from build123d import *

# Parameters (mm, degrees)
F0_W         = 100
F0_H         = 40
F1_DEPTH     = 10
F3_DEPTH     = 8.82827
F4_W         = 40
F4_H         = 3
F5_DEPTH     = 40.001
F6_R         = 2.25
F7_DEPTH     = 40.001
F8_R         = 4.5
F9_DEPTH     = 5.7
F10_T1_DEPTH = 40
F10_T3_DEPTH = 50
F10_T5_DEPTH = 50
F10_T7_DEPTH = 50
F10_T9_DEPTH = 50
F11_T1_DEPTH = 40
F12_R        = 3


# Not quite as in the source:
# - a fillet or chamfer that OpenCascade refuses, or shapes differently, is made with other operations: its cross-section is extruded or revolved along the edge and cut away or added


with BuildPart() as f1:
    # F0 (on Top) → F1 (new body)
    with BuildSketch(Plane.XY):
        with Locations((-50, 20)):
            Rectangle(F0_W, F0_H)
    extrude(amount=F1_DEPTH)

    # F2 (on face) → F3 (join)
    with BuildSketch(Plane.XZ):
        with BuildLine():
            ThreePointArc((-30, 35), (-50, 55), (-70, 35))
            Line((-70, 35), (-70, 0))
            Line((-70, 0), (-30, 0))
            Line((-30, 0), (-30, 35))
        make_face()
    extrude(amount=-F3_DEPTH)

    # F4 (on Front) → F5 (cut, through all)
    with BuildSketch(Plane.XZ):
        with Locations((-50, 1.5)):
            Rectangle(F4_W, F4_H)
    extrude(amount=-F5_DEPTH, mode=Mode.SUBTRACT)

    # F6 (on face) → F7 (cut, through all)
    with BuildSketch(Plane.XZ):
        with Locations((-50, 35)):
            Circle(F6_R)
    extrude(amount=-F7_DEPTH, mode=Mode.SUBTRACT)

    # F8 (on face) → F9 (cut)
    with BuildSketch(Plane.XZ):
        with Locations((-50, 35)):
            Circle(F8_R)
    extrude(amount=-F9_DEPTH, mode=Mode.SUBTRACT)

    # F10: fillet of radius 8 on 5 edges, made by hand

    # F10_s2 → F10_t1 (join)
    with BuildSketch(Plane.XZ.offset(-40)):
        with BuildLine():
            ThreePointArc((-36.2449979984, 3), (-32.7808963833, 2.2111025509), (-30, 0))
            Line((-30, 0), (-30, 3))
            Line((-30, 3), (-36.2449979984, 3))
        make_face()
    extrude(amount=F10_T1_DEPTH)

    # F10_s4 → F10_t3 (cut)
    with BuildSketch(Plane.XY.offset(-20)):
        with BuildLine():
            ThreePointArc((-92, 0), (-97.6568542495, 2.3431457505), (-100, 8))
            Line((-100, 8), (-100, 0))
            Line((-100, 0), (-92, 0))
        make_face()
    extrude(amount=F10_T3_DEPTH, mode=Mode.SUBTRACT)

    # F10_s6 → F10_t5 (cut)
    with BuildSketch(Plane.XY.offset(-20)):
        with BuildLine():
            ThreePointArc((-8, 0), (-2.3431457505, 2.3431457505), (0, 8))
            Line((0, 8), (0, 0))
            Line((0, 0), (-8, 0))
        make_face()
    extrude(amount=F10_T5_DEPTH, mode=Mode.SUBTRACT)

    # F10_s8 → F10_t7 (cut)
    with BuildSketch(Plane.XY.offset(-20)):
        with BuildLine():
            ThreePointArc((-100, 32), (-97.6568542495, 37.6568542495), (-92, 40))
            Line((-92, 40), (-100, 40))
            Line((-100, 40), (-100, 32))
        make_face()
    extrude(amount=F10_T7_DEPTH, mode=Mode.SUBTRACT)

    # F10_s10 → F10_t9 (cut)
    with BuildSketch(Plane.XY.offset(-20)):
        with BuildLine():
            ThreePointArc((-8, 40), (-2.3431457505, 37.6568542495), (0, 32))
            Line((0, 32), (0, 40))
            Line((0, 40), (-8, 40))
        make_face()
    extrude(amount=F10_T9_DEPTH, mode=Mode.SUBTRACT)

    # F11: fillet of radius 8 on 1 edges, made by hand

    # F11_s2 → F11_t1 (join)
    with BuildSketch(Plane.XZ.offset(-40)):
        with BuildLine():
            ThreePointArc((-70, 0), (-67.2191036167, 2.2111025509), (-63.7550020016, 3))
            Line((-63.7550020016, 3), (-70, 3))
            Line((-70, 3), (-70, 0))
        make_face()
    extrude(amount=F11_T1_DEPTH)

    # F12
    f12_edges = [f1.edges().sort_by_distance(p)[0] for p in [
        (-50, 8.82827, 55),
        (-30, 8.82827, 22.5),
        (-70, 8.82827, 22.5),
    ]]
    fillet(f12_edges, radius=F12_R)


solid = f1.part
Input: part model. Units: mm. Frame: model coordinates. A direction names the side the tool comes from. Give positions to 0.01 mm unless a question says otherwise; leave off trailing zeros. Write each loop counter-clockwise with the first axis right and the second up, starting at its lowest first coordinate (ties: lowest second). Pieces come first, ordered by that corner, then holes.
Q1. Material intervals for probe 1 along Z at (x, y) = (-50, 2.1); probe 2 along Z at (x, y) = (-90, 35.5); probe 3 along Y at (x, z) = (-51.5, 37), sorted ascending.
Q2. First-contact query: P1, Ø1, axis at y = 4.5, z = 27.5, coming from the +X side; P2, Ø6.5, axis at y = 4, z = 19.5, coming from the -X side; P3, Ø1.5, axis at x = -15, y = 11, coming from the +Z side; P4, Ø7, axis at x = -50.5, z = 34, coming from the -Y side. Flat tips, straight axial feed; report the tip coordinate or a pass-through.
Q3. Section C-C, the plane y = 3.5. Output: boundary loops of the cut face in (x, z) (3 decimals), plus the area to 3 significant figures.
Q4. Section D-D, the plane x = -87.5. Output: boundary loops of the cut face in (y, z).
Q5. Set-up query: faces 1 (the face through (-47.92, 2.81, 31.01)), 2 (the face through (-30, 3, 22)), 3 (the face through (-69.14, 7.93, 22.32)), 4 (the face through (-50, 8.828, 31)). Return all of +Z, -Z, +X, -X, +Y, -Y with unobstructed straight access to the full face (end or side cutting, diameter ignored); none if empty.
Q6. Pull-direction query (X, two-part tool) for faces 5 (the face through (-51, 40, 5)), 6 (the face through (-50, 20, 3)), 7 (the face through (-30.86, 7.93, 22.68)), 8 (the face through (-48, 5.7, 33)); classes: pulls with the +X half, pulls with the -X half, needs draft (parallel to the pull), parting line crosses it, or undercut.
Q7. Section A-A, the plane x = -50. Output: boundary loops of the cut face in (y, z).
Q8. Section B-B, the plane y = 22.5. Output: boundary loops of the cut face in (x, z) (3 decimals).
Filled in:
1. probe 1: z = 3 to 30.5, 39.5 to 55
1. probe 2: z = 0 to 10
1. probe 3: y = 5.7 to 8.83
2. P1: stops at x = -30
2. P2: stops at x = -70
2. P3: stops at z = 10
2. P4: stops at y = 0
3. outline: (-98.614, 0) - (-70, 0) arc R8 cw to (-63.755, 3) - (-36.245, 3) arc R8 cw to (-30, 0) - (-1.386, 0) - (-1.386, 10) - (-30, 10) - (-30, 35) arc R20 ccw to (-70, 35) - (-70, 10) - (-98.614, 10) - close; hole circle Ø9 at (-50, 35)
3. area: 2,430 mm2
4. outline: (0, 0) - (40, 0) - (40, 10) - (0, 10) - close
5. face 1: -Y
5. face 2: +Z, +X, +Y, -Y
5. face 3: +Z, -X, +Y
5. face 4: +Z, +X, -X, +Y
6. face 5: needs draft
6. face 6: undercut
6. face 7: pulls with the +X half
6. face 8: undercut
7. outline: (0, 3) - (40, 3) - (40, 10) - (8.83, 10) - (8.83, 32.75) - (5.7, 32.75) - (5.7, 30.5) - (0, 30.5) - close; (0, 39.5) - (5.7, 39.5) - (5.7, 37.25) - (8.83, 37.25) - (8.83, 52) arc R3 ccw to (5.83, 55) - (0, 55) - close
8. outline: (-100, 0) - (-70, 0) arc R8 cw to (-63.755, 3) - (-36.245, 3) arc R8 cw to (-30, 0) - (0, 0) - (0, 10) - (-100, 10) - close
